For this review, take the finished solid that the model builds, in its own axes (mm). Round coordinates to 2 decimals unless told otherwise and drop trailing zeros. Write each loop counter-clockwise with the first axis right and the second up, starting at its lowest first coordinate (ties: lowest second). Pieces come first, ordered by that corner, then holes. Notation, with made-up numbers: (62.25, 65.25) -> (96.25, 65.25) arc R15 ccw to (96.25, 73.25) -> close; hole circle Ø3 at (-37.5, 26). An arc over 180 degrees is marked (long way). Answer in a Markdown table with one row per item.
from build123d import *

# Parameters (mm, degrees)
SKETCH1_R           = 3
BOSS_EXTRUDE1_DEPTH = 3


with BuildPart() as part:
    # Sketch1 → Boss-Extrude1 (new body)
    # profile 1 of 7: a face of its own
    with BuildSketch(Plane.XY):
        with BuildLine():
            ThreePointArc((1328.13150473, -1693.072432874), (1328.496972448, -1691.186259901), (1328.13150473, -1689.300086927))
            Line((1328.13150473, -1689.300086927), (1327.422718332, -1688.072432874))
            ThreePointArc((1327.422718332, -1688.072432874), (1325.97197848, -1686.812842059), (1324.15577091, -1686.186259901))
            Line((1324.15577091, -1686.186259901), (1322.738198114, -1686.186259901))
            ThreePointArc((1322.738198114, -1686.186259901), (1320.921990544, -1686.812842059), (1319.471250692, -1688.072432874))
            Line((1319.471250692, -1688.072432874), (1318.762464294, -1689.300086927))
            ThreePointArc((1318.762464294, -1689.300086927), (1318.396996575, -1691.186259901), (1318.762464294, -1693.072432874))
            Line((1318.762464294, -1693.072432874), (1319.471250692, -1694.300086927))
            ThreePointArc((1319.471250692, -1694.300086927), (1320.921990544, -1695.559677742), (1322.738198114, -1696.186259901))
            Line((1322.738198114, -1696.186259901), (1324.15577091, -1696.186259901))
            ThreePointArc((1324.15577091, -1696.186259901), (1325.97197848, -1695.559677742), (1327.422718332, -1694.300086927))
            Line((1327.422718332, -1694.300086927), (1328.13150473, -1693.072432874))
        make_face()
        with Locations((1323.446984512, -1691.186259901)):
            Circle(SKETCH1_R, mode=Mode.SUBTRACT)
    # profile 2 of 7: a face of its own
    with BuildSketch(Plane.XY):
        with BuildLine():
            Line((1321.752495925, -1695.943474063), (1324.499074459, -1696.921787568))
            Line((1324.499074459, -1696.921787568), (1326.719608123, -1695.032337494))
            ThreePointArc((1326.719608123, -1695.032337494), (1325.519613433, -1695.791320976), (1324.15577091, -1696.186259901))
            Line((1324.15577091, -1696.186259901), (1322.738198114, -1696.186259901))
            ThreePointArc((1322.738198114, -1696.186259901), (1322.239230852, -1696.089698414), (1321.752495925, -1695.943474063))
        make_face()
    # profile 3 of 7: a face of its own
    with BuildSketch(Plane.XY):
        with BuildLine():
            ThreePointArc((1327.422718332, -1694.300086927), (1327.089609813, -1694.683924703), (1326.719608123, -1695.032337494))
            Line((1326.719608123, -1695.032337494), (1328.940142149, -1693.142887113))
            Line((1328.940142149, -1693.142887113), (1328.414095669, -1690.275115064))
            ThreePointArc((1328.414095669, -1690.275115064), (1328.471399282, -1691.693836867), (1328.13150473, -1693.072432874))
            Line((1328.13150473, -1693.072432874), (1327.422718332, -1694.300086927))
        make_face()
    # profile 4 of 7: a face of its own
    with BuildSketch(Plane.XY):
        with BuildLine():
            ThreePointArc((1328.13150473, -1689.300086927), (1328.29736254, -1689.780482129), (1328.414095669, -1690.275115064))
            Line((1328.414095669, -1690.275115064), (1327.888052202, -1687.407359446))
            Line((1327.888052202, -1687.407359446), (1325.141464891, -1686.429042814))
            ThreePointArc((1325.141464891, -1686.429042814), (1326.398766175, -1687.08877736), (1327.422718332, -1688.072432874))
            Line((1327.422718332, -1688.072432874), (1328.13150473, -1689.300086927))
        make_face()
    # profile 5 of 7: a face of its own
    with BuildSketch(Plane.XY):
        with BuildLine():
            ThreePointArc((1324.15577091, -1686.186259901), (1324.654733942, -1686.282820345), (1325.141464891, -1686.429042814))
            Line((1325.141464891, -1686.429042814), (1322.394894565, -1685.450732233))
            Line((1322.394894565, -1685.450732233), (1320.17435296, -1687.340189064))
            ThreePointArc((1320.17435296, -1687.340189064), (1321.374350836, -1686.581200964), (1322.738198114, -1686.186259901))
            Line((1322.738198114, -1686.186259901), (1324.15577091, -1686.186259901))
        make_face()
    # profile 6 of 7: a face of its own
    with BuildSketch(Plane.XY):
        with BuildLine():
            Line((1317.953826874, -1689.229632688), (1318.479872929, -1692.097402415))
            ThreePointArc((1318.479872929, -1692.097402415), (1318.42256986, -1690.67868176), (1318.762464294, -1689.300086927))
            Line((1318.762464294, -1689.300086927), (1319.471250692, -1688.072432874))
            ThreePointArc((1319.471250692, -1688.072432874), (1319.8043556, -1687.688598858), (1320.17435296, -1687.340189064))
            Line((1320.17435296, -1687.340189064), (1317.953826874, -1689.229632688))
        make_face()
    # profile 7 of 7: a face of its own
    with BuildSketch(Plane.XY):
        with BuildLine():
            Line((1319.005916822, -1694.965160355), (1321.752495925, -1695.943474063))
            ThreePointArc((1321.752495925, -1695.943474063), (1320.495199314, -1695.283739895), (1319.471250692, -1694.300086927))
            Line((1319.471250692, -1694.300086927), (1318.762464294, -1693.072432874))
            ThreePointArc((1318.762464294, -1693.072432874), (1318.596606155, -1692.592036538), (1318.479872929, -1692.097402415))
            Line((1318.479872929, -1692.097402415), (1319.005916822, -1694.965160355))
        make_face()
    extrude(amount=-BOSS_EXTRUDE1_DEPTH)


solid = part.part
1) Consider section C-C on z = -1.4. State the section outline as (x, y) points.
Solved:
| item | result |
|---|---|
| outline | (1317.95, -1689.23) -> (1319.01, -1694.97) -> (1324.5, -1696.92) -> (1328.94, -1693.14) -> (1327.89, -1687.41) -> (1322.39, -1685.45) -> close; hole circle Ø6 at (1323.45, -1691.19) |
2) Consider section B-B on x = 1323. State the section outline as (y, z) points, then the cut area to 3 significant figures.
Solved:
| item | result |
|---|---|
| outline | (-1696.39, -3) -> (-1694.15, -3) -> (-1694.15, 0) -> (-1696.39, 0) -> close; (-1688.22, -3) -> (-1685.67, -3) -> (-1685.67, 0) -> (-1688.22, 0) -> close |
| area | 14.4 mm² |
3) Mouldability with a two-part tool opening along X and no side actions: class faces 1 (the flat face through (1326, -1694, 0)), 2 (the cylindrical face through (1321.066, -1693.012, -1.479)) as pulls with the +X half, pulls with the -X half, needs draft (parallel to the pull), parting line crosses it, or undercut.
Solved:
| item | result |
|---|---|
| face 1 | needs draft |
| face 2 | undercut |
4) For line 1 (X direction, y = -1690, z = -0.5); line 2 (Y direction, x = 1323.25, z = -2.75); line 3 (X direction, y = -1692.75, z = -1.6), list the stretches that pass through material, from the lowest coordinate up. Write a range as [from, to].
Solved:
| item | result |
|---|---|
| line 1 | [1318.1, 1320.69], [1326.2, 1328.36] |
| line 2 | [-1696.48, -1694.18], [-1688.19, -1685.76] |
| line 3 | [1318.6, 1320.89], [1326.01, 1328.87] |
5) Consider section D-D on y = -1686.75. State the section outline as (x, z) points.
Solved:
| item | result |
|---|---|
| outline | (1320.87, -3) -> (1326.04, -3) -> (1326.04, 0) -> (1320.87, 0) -> close |
6) Consider section A-A on y = -1692.5. State the section outline as (x, z) points, then the cut area to 3 significant figures.
Solved:
| item | result |
|---|---|
| outline | (1318.55, -3) -> (1320.75, -3) -> (1320.75, 0) -> (1318.55, 0) -> close; (1326.14, -3) -> (1328.82, -3) -> (1328.82, 0) -> (1326.14, 0) -> close |
| area | 14.6 mm² |
